Can you work these out from the model? Positions are in its coordinate system, mm. A direction names the side the tool comes from. Round coordinates to 2 decimals unless told otherwise and drop trailing zeros. Loops run counter-clockwise (first coordinate to the right, second up) from the corner with the lowest first, then second, coordinate; pieces in that order, holes last.
Autodesk Inventor part; units mm, degrees
ref_plane "YZ Plane" through (0, 0, 0) normal (1, 0, 0) x (0, 1, 0)
ref_plane "XZ Plane" through (0, 0, 0) normal (0, 1, 0) x (-1, 0, 0)
ref_plane "XY Plane" through (0, 0, 0) normal (0, 0, 1) x (1, 0, 0)
sketch "スケッチ1" plane through (0, 0, 0) normal (0, 0, 1) x (1, 0, 0)
  line L0 (-26, 18) -> (26, 18)
  line L1 (26, 18) -> (26, -18)
  line L2 (26, -18) -> (-26, -18)
  line L3 (-26, -18) -> (-26, 18)
  point P0 (0, 0)
  point P1 (0, -18)
  point P2 (-26, 0)
  dimension "d0" = 52
  dimension "d1" = 36
extrude "押し出し1" add sketch "スケッチ1" along normal blind 10
sketch "スケッチ2" plane through (0, 0, 10) normal (0, 0, 1) x (1, 0, 0)
  line L0 (-26, 18) -> (26, 18)
  line L1 (26, -18) -> (-26, -18)
  line L2 (-15, 18) -> (15, 18)
  line L3 (15, 18) -> (15, -18)
  line L4 (15, -18) -> (-15, -18)
  line L5 (-15, -18) -> (-15, 18)
  point P0 (0, 0)
  point P1 (0, -18)
  point P2 (0, -18)
  dimension "d4" = 30
extrude "押し出し2" add sketch "スケッチ2" along normal blind 30
sketch "スケッチ3" plane through (0, 0, 40) normal (0, 0, 1) x (1, 0, 0)
  line L0 (15, -18) -> (-15, -18)
  line L1 (-10, 13) -> (10, 13)
  line L2 (10, 13) -> (10, -7)
  line L3 (10, -7) -> (-10, -7)
  line L4 (-10, -7) -> (-10, 13)
  point P0 (0, 0)
  point P1 (0, -7)
  dimension "d7" = 20
  dimension "d8" = 20
  dimension "d9" = 11
extrude "押し出し3" cut sketch "スケッチ3" against normal through all
sketch "スケッチ4" plane through (0, 0, 10) normal (0, 0, 1) x (1, 0, 0)
  point P0 (0, 0)
  point P1 (-21, -12)
  dimension "d12" = 12
  dimension "d13" = 21
hole "穴1" at (-21, -12, 10) direction (0, 0, -1) diameter 5.5 end through all
pattern_linear "矩形状パターン1" count 2 spacing 42 along (1, 0, 0) count 2 spacing 24 along (0, 1, 0) of "穴1"
sketch "スケッチ5" plane through (-26, -18, 0) normal (0, -1, 0) x (1, 0, 0)
  line L0 (41, 10) -> (41, 40)
  line L1 (41, 40) -> (11, 40)
  line L2 (11, 10) -> (11, 40)
  line L3 (52, 0) -> (0, 0)
  line L4 (11, 14) -> (41, 14)
  line L5 (41, 14) -> (41, 12)
  line L6 (41, 12) -> (11, 12)
  line L7 (11, 12) -> (11, 14)
  line L8 (25, 40) -> (27, 40)
  line L9 (27, 40) -> (27, 11.5)
  line L10 (27, 11.5) -> (25, 11.5)
  line L11 (25, 11.5) -> (25, 40)
  point P0 (26, 0)
  point P1 (26, 11.5)
  point P2 (26, 0)
  dimension "d27" = 12
  dimension "d28" = 2
  dimension "d29" = 2
  dimension "d30" = 0.5
extrude "押し出し4" cut sketch "スケッチ5" against normal up to surface (11 mm away) contours L6 L9 L4 L0 | L9 L10 L11 L6 | L6 L11 L4 L9 | L4 L11 L1 L9 | L6 L2 L4 L11
sketch "スケッチ6" plane through (-15, -7, 14) normal (0, -1, 0) x (1, 0, 0)
  line L0 (5, 0) -> (5, -2)
  line L1 (0, 0) -> (5, 0)
  line L2 (0, -2) -> (0, 0)
  line L3 (5, -2) -> (0, -2)
  line L4 (25, 0) -> (25, -2)
  line L5 (30, -2) -> (25, -2)
  line L6 (30, 0) -> (30, -2)
  line L7 (25, 0) -> (30, 0)
  point P0 (15, -14)
extrude "押し出し5" cut sketch "スケッチ6" against normal up to surface (20 mm away)
sketch "スケッチ7" plane through (15, -18, 10) normal (1, 0, 0) x (0, 0, -1)
  line L0 (-4, 0) -> (-30, 0)
  line L1 (10, 36) -> (10, 0)
  point P0 (10, 18)
  point P1 (-16.5, 6)
  dimension "d35" = 26.5
  dimension "d36" = 6
hole "穴2" at (15, -12, 26.5) direction (-1, 0, 0) diameter 5.5 end up to surface counterbore diameter 9.5 counterbore depth 5.5
sketch "スケッチ8" plane through (-15, -18, 10) normal (-1, 0, 0) x (0, 0, 1)
  circle A0 centre (16.5, 6) radius 2.75
  point P0 (-10, 18)
hole "穴3" at (-15, -12, 26.5) direction (1, 0, 0) diameter 4.134 end up to surface
chamfer "面取り1" distance 1 angle 45 4 edges at (-26, 18, 5) (-26, -18, 5) (26, 18, 5) (26, -18, 5)
equation "\"d8\" = d7"
properties part number "CLQAM20" material "MISUMI"
(1) For pin 1 (3.5 mm diameter, centred on y = -12.5, z = 26.5, fed in from -X); pin 2 (3.5 mm diameter, centred on x = -18.5, y = 4.5, fed in from +Z); pin 3 (3.5 mm diameter, centred on y = -12, z = 26.5, fed in from +X); pin 4 (12 mm diameter, centred on y = -14.5, z = 20.5, fed in from +X), each with a flat end and sliding along its axis, tell me the tip position at first contact or that it passes through.
(2) If I drill on line 1 (Z direction, x = 13.1, y = -12); line 2 (X direction, y = 12, z = 7); line 3 (Y direction, x = -21, z = 7.5), over which ranges is the centre line in solid material (lowest first)?
(3) We'd pull the mould along Y, two halves only. Please class faces 5 (the flat face through (0, -7, 6)), 6 (the flat face through (0, 18, 15)), 7 (the flat face through (-8, -18, 27)), 8 (the flat face through (-11, -6, 14)): released by +Y, released by -Y, zero draft, split by the parting line, or undercut.
(4) Suppose I cut it at C-C (z = 26.5). Write out the boundary of the cut face in (x, y).
(5) Suppose I cut it at D-D (x = 21). Write out the boundary of the cut face in (y, z), then the cut area to 3 significant figures.
(6) Suppose I cut it at B-B (y = 3). Write out the boundary of the cut face in (x, z).
(7) Suppose I cut it at A-A (x = -7). Write out the boundary of the cut face in (y, z), then the cut area to 3 significant figures.
(8) Which directions (+Z, -Z, +X, -X, +Y, -Y) give clear straight access to the entire face, cutting with the end or side of a thin tool? Please do faces 1 (the flat face through (26, 0, 5)), 2 (the flat face through (1, -15, 27)), 3 (the flat face through (15, 0, 25)), 4 (the flat face through (-10, 3, 6)).
Check result:
1. pin 1: stops at x = -15
1. pin 2: stops at z = 10
1. pin 3: passes through
1. pin 4: stops at x = 15
2. line 1: z = 0 to 12, 14 to 21.75, 31.25 to 40
2. line 2: x = -26 to -23.75, -18.25 to -10, 10 to 18.25, 23.75 to 26
2. line 3: y = -18 to -14.75, -9.25 to 9.25, 14.75 to 18
3. face 5: undercut
3. face 6: released by +Y
3. face 7: released by -Y
3. face 8: zero draft
4. outline: (-15, -18) - (-1, -18) - (-1, -14.07) - (-15, -14.07) - close; (-15, -9.93) - (-1, -9.93) - (-1, -7) - (-10, -7) - (-10, 13) - (10, 13) - (10, -7) - (1, -7) - (1, -9.25) - (9.5, -9.25) - (9.5, -7.25) - (15, -7.25) - (15, 18) - (-15, 18) - close; (1, -18) - (15, -18) - (15, -16.75) - (9.5, -16.75) - (9.5, -14.75) - (1, -14.75) - close
5. outline: (-18, 0) - (-14.75, 0) - (-14.75, 10) - (-18, 10) - close; (-9.25, 0) - (9.25, 0) - (9.25, 10) - (-9.25, 10) - close; (14.75, 0) - (18, 0) - (18, 10) - (14.75, 10) - close
5. area: 250 mm2
6. outline: (-26, 0) - (-10, 0) - (-10, 12) - (-15, 12) - (-15, 10) - (-26, 10) - close; (-15, 14) - (-10, 14) - (-10, 40) - (-15, 40) - close; (10, 0) - (26, 0) - (26, 10) - (15, 10) - (15, 12) - (10, 12) - close; (10, 14) - (15, 14) - (15, 40) - (10, 40) - close
7. outline: (-18, 0) - (-7, 0) - (-7, 12) - (-18, 12) - close; (-18, 14) - (-7, 14) - (-7, 40) - (-18, 40) - close; (13, 0) - (18, 0) - (18, 40) - (13, 40) - close; hole circle Ø4.13 at (-12, 26.5)
7. area: 605 mm2
8. face 1: +Z, -Z, +X, +Y, -Y
8. face 2: +Z, -Y
8. face 3: +Z, +X, +Y, -Y
8. face 4: +Z, -Z
